For this review, take the finished solid that the model builds, in its own axes (mm). Face numbers are marked on the shaded views. A direction names the side the tool comes from. Round coordinates to 2 decimals unless told otherwise and drop trailing zeros. Write each loop counter-clockwise with the first axis right and the second up, starting at its lowest first coordinate (ties: lowest second). Pieces come first, ordered by that corner, then holes. Notation, with made-up numbers: M -31.75,-11.5 L 18.25,-11.5 A26 ccw 18.25,14.5 Z; hole C -20.75,6 d11. An arc over 180 degrees is marked long. One line per question, with ' | ' between items.
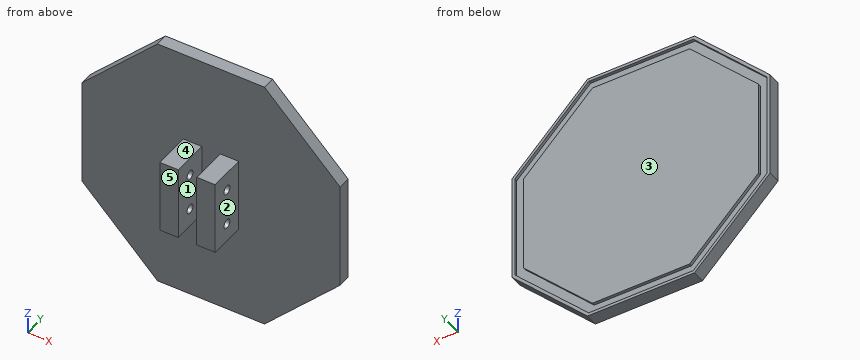
Autodesk Inventor part; units mm, degrees
ref_plane "YZ Plane" through (0, 0, 0) normal (1, 0, 0) x (0, 1, 0)
ref_plane "XZ Plane" through (0, 0, 0) normal (0, 1, 0) x (-1, 0, 0)
ref_plane "XY Plane" through (0, 0, 0) normal (0, 0, 1) x (1, 0, 0)
sketch "스케치3" plane through (0, 0, 0) normal (0, 1, 0) x (-1, 0, 0)
  line L0 (34.9919, -14.4941) -> (14.4941, -34.9919)
  line L1 (14.4941, -34.9919) -> (-14.4941, -34.9919)
  line L2 (-14.4941, -34.9919) -> (-34.9919, -14.4941)
  line L3 (-34.9919, -14.4941) -> (-34.9919, 14.4941)
  line L4 (-34.9919, 14.4941) -> (-14.4941, 34.9919)
  line L5 (-14.4941, 34.9919) -> (14.4941, 34.9919)
  line L6 (14.4941, 34.9919) -> (34.9919, 14.4941)
  line L7 (34.9919, 14.4941) -> (34.9919, -14.4941)
  line L8 (13.5, -32.5919) -> (-13.5, -32.5919)
  line L9 (-13.5, -32.5919) -> (-32.5919, -13.5)
  line L10 (-32.5919, -13.5) -> (-32.5919, 13.5)
  line L11 (-32.5919, 13.5) -> (-13.5, 32.5919)
  line L12 (-13.5, 32.5919) -> (13.5, 32.5919)
  line L13 (13.5, 32.5919) -> (32.5919, 13.5)
  line L14 (32.5919, 13.5) -> (32.5919, -13.5)
  line L15 (32.5919, -13.5) -> (13.5, -32.5919)
  point P0 (0, 0)
  point P1 (0, 0)
  point P2 (0, 0)
  point P3 (0, 0)
  dimension "d66" = 27
  dimension "d67" = 2.4
extrude "돌출2" add sketch "스케치3" along normal blind 3.4 contours L0 L1 L2 L3 L4 L5 L6 L7 | L8 L9 L10 L11 L12 L13 L14 L15
sketch "스케치4" plane through (0, 3.4, 0) normal (0, 1, 0) x (1, 0, 0)
  line L0 (13.5, -32.5919) -> (-13.5, -32.5919)
  line L1 (-13.5, -32.5919) -> (-32.5919, -13.5)
  line L2 (-32.5919, -13.5) -> (-32.5919, 13.5)
  line L3 (-32.5919, 13.5) -> (-13.5, 32.5919)
  line L4 (-13.5, 32.5919) -> (13.5, 32.5919)
  line L5 (13.5, 32.5919) -> (32.5919, 13.5)
  line L6 (32.5919, 13.5) -> (32.5919, -13.5)
  line L7 (32.5919, -13.5) -> (13.5, -32.5919)
  line L8 (-14.1627, 34.1919) -> (14.1627, 34.1919)
  line L9 (14.1627, 34.1919) -> (34.1919, 14.1627)
  line L10 (34.1919, 14.1627) -> (34.1919, -14.1627)
  line L11 (34.1919, -14.1627) -> (14.1627, -34.1919)
  line L12 (14.1627, -34.1919) -> (-14.1627, -34.1919)
  line L13 (-14.1627, -34.1919) -> (-34.1919, -14.1627)
  line L14 (-34.1919, -14.1627) -> (-34.1919, 14.1627)
  line L15 (-34.1919, 14.1627) -> (-14.1627, 34.1919)
  line L16 (-13.1686, 31.7919) -> (13.1686, 31.7919)
  line L17 (13.1686, 31.7919) -> (31.7919, 13.1686)
  line L18 (31.7919, 13.1686) -> (31.7919, -13.1686)
  line L19 (31.7919, -13.1686) -> (13.1686, -31.7919)
  line L20 (13.1686, -31.7919) -> (-13.1686, -31.7919)
  line L21 (-13.1686, -31.7919) -> (-31.7919, -13.1686)
  line L22 (-31.7919, -13.1686) -> (-31.7919, 13.1686)
  line L23 (-31.7919, 13.1686) -> (-13.1686, 31.7919)
  point P0 (0, 0)
  point P1 (0, 0)
  point P2 (0, 0)
  point P3 (0, 0)
  dimension "d7" = 27
  dimension "d68" = 1.6
  dimension "d69" = 0.8
extrude "돌출3" cut sketch "스케치4" against normal blind 0.8 contours L0 L1 L2 L3 L4 L5 L6 L7 | L8 L9 L10 L11 L12 L13 L14 L15
sketch "스케치9" plane through (0, 0, 0) normal (0, -1, 0) x (1, 0, 0)
  line L0 (7.5, 10) -> (2.5, 10)
  line L1 (2.5, 10) -> (2.5, -10)
  line L2 (2.5, -10) -> (7.5, -10)
  line L3 (7.5, -10) -> (7.5, 10)
  line L4 (7.5, 10) -> (2.5, -10) construction
  line L5 (2.5, 10) -> (7.5, -10) construction
  line L6 (-2.5, 10) -> (-7.5, 10)
  line L7 (-7.5, 10) -> (-7.5, -10)
  line L8 (-7.5, -10) -> (-2.5, -10)
  line L9 (-2.5, 10) -> (-7.5, -10) construction
  line L10 (-7.5, 10) -> (-2.5, -10) construction
  line L11 (-2.5, -10) -> (-2.5, 10)
  point P0 (0, 0)
  point P1 (5, 0)
  point P2 (-5, 0)
  dimension "d42" = 20
  dimension "d43" = 5
  dimension "d44" = 2.5
  dimension "d47" = 10
extrude "돌출8" add sketch "스케치9" along normal blind 10
sketch "스케치10" plane through (-7.5, 0, -10) normal (-1, 0, 0) x (0, 0, 1)
  circle A0 centre (15, -5) radius 1.25
  line L0 (19.9591, 0) -> (0.0886, 0)
  line L1 (24.4941, 0) -> (-4.4941, 0)
  circle A1 centre (5, -5) radius 1.25
  line L2 (20, 0) -> (20, -10)
  point P0 (10, 0)
  dimension "d54" = 2.5
  dimension "d57" = 10
  dimension "d62" = 5
  dimension "d63" = 5
extrude "돌출9" cut sketch "스케치10" against normal blind 20
properties part number "팔각형 OV-PAM 5패턴 하단 - 틈 너비 수정"
Item 1: To check wall thickness, follow line 1 along Y through (x, z) = (-5.5, -5); line 2 along X through (y, z) = (-1.25, -8.5); line 3 along Y through (x, z) = (30, 12.5). State the ranges of each line that lie inside material, in increasing order. Write a range as from..to.
Results:
line 1: -10..-6.25, -3.75..3.4 | line 2: -7.5..-2.5, 2.5..7.5 | line 3: 0..3.4
Item 2: Take a section at D-D (z = -8). Write out the cut boundary in (x, y).
Results:
outline: M -34.99,0 L -7.5,0 L -7.5,-10 L -2.5,-10 L -2.5,0 L 2.5,0 L 2.5,-10 L 7.5,-10 L 7.5,0 L 34.99,0 L 34.99,3.4 L 34.19,3.4 L 34.19,2.6 L 31.79,2.6 L 31.79,3.4 L -31.79,3.4 L -31.79,2.6 L -34.19,2.6 L -34.19,3.4 L -34.99,3.4 Z
Item 3: Take a section at C-C (x = -6.5). Write out the cut boundary in (y, z), then the cut area to 3 significant figures.
Results:
outline: M -10,-10 L 0,-10 L 0,-34.99 L 3.4,-34.99 L 3.4,-34.19 L 2.6,-34.19 L 2.6,-31.79 L 3.4,-31.79 L 3.4,31.79 L 2.6,31.79 L 2.6,34.19 L 3.4,34.19 L 3.4,34.99 L 0,34.99 L 0,10 L -10,10 Z; hole C -5,-5 d2.5; hole C -5,5 d2.5 | area: 424 mm2
Item 4: Take a section at A-A (y = -5). Write out the cut boundary in (x, z), then the cut area to 3 significant figures.
Results:
outline: M -7.5,-10 L -2.5,-10 L -2.5,-6.25 L -7.5,-6.25 Z; M -7.5,-3.75 L -2.5,-3.75 L -2.5,3.75 L -7.5,3.75 Z; M -7.5,6.25 L -2.5,6.25 L -2.5,10 L -7.5,10 Z; M 2.5,-10 L 7.5,-10 L 7.5,-6.25 L 2.5,-6.25 Z; M 2.5,-3.75 L 7.5,-3.75 L 7.5,3.75 L 2.5,3.75 Z; M 2.5,6.25 L 7.5,6.25 L 7.5,10 L 2.5,10 Z | area: 150 mm2
Item 5: Insertion check: pin 1 Ø1 at (y, z) = (-5, 11.5) entering from -X (1 decimal); pin 2 Ø3 at (y, z) = (-5, 5) entering from +X; pin 3 Ø2 at (y, z) = (-2.5, 3.5) entering from -X; pin 4 Ø12 at (x, z) = (-19, 2.5) entering from -Y. Each pin has a flat end and moves straight along its axis. Give the tip position at first contact, or say it passes through.
Results:
pin 1: through | pin 2: x = 7.5 | pin 3: x = -7.5 | pin 4: y = 0
Item 6: Machinability: for the marked faces 4 and 5, which of the approach directions +Z, -Z, +X, -X, +Y, -Y give a long, thin tool a straight path to every point of the face, cutting with its end or side? Answer none if there is none.
Results:
face 4: +Z, +X, -X, -Y | face 5: +Z, -Z, +X, -X, -Y
Item 7: Mouldability with a two-part tool opening along X and no side actions: class the marked faces 1, 2 and 3 as +X half, -X half, draft (parallel to the pull), parting line (faces both ways), or undercut.
Results:
face 1: undercut | face 2: +X half | face 3: draft
Item 8: Take a section at B-B (z = 5). Write out the cut boundary in (x, y), then the cut area to 3 significant figures.
Results:
outline: M -34.99,0 L -7.5,0 L -7.5,-3.75 L -2.5,-3.75 L -2.5,0 L 2.5,0 L 2.5,-3.75 L 7.5,-3.75 L 7.5,0 L 34.99,0 L 34.99,3.4 L 34.19,3.4 L 34.19,2.6 L 31.79,2.6 L 31.79,3.4 L -31.79,3.4 L -31.79,2.6 L -34.19,2.6 L -34.19,3.4 L -34.99,3.4 Z; M -7.5,-10 L -2.5,-10 L -2.5,-6.25 L -7.5,-6.25 Z; M 2.5,-10 L 7.5,-10 L 7.5,-6.25 L 2.5,-6.25 Z | area: 309 mm2
